Read the model definition and answer for the solid it produces. Units are mm, in the model's axes. A direction names the side the tool comes from. Give positions to 0.01 mm unless a question says otherwise; leave off trailing zeros. Order: outer loops, then holes, each group sorted by start corner. A loop starts at its lowest first (then second) coordinate and runs counter-clockwise, first axis right, second up. Notation, with made-up numbers: M 46,-39 L 75,-39 A12 cw 75,-32 Z; hole C 66.5,33 d7. An arc over 180 degrees is marked long. One line per item, written item: value.
from build123d import *

# Parameters (mm, degrees)
SKETCH_1_R          = 1.5
EXTRUDE_2_DEPTH     = 3
SKETCH_2_R          = 1.5
CUT_EXTRUDE_1_DEPTH = 10
CUT_EXTRUDE_2_DEPTH = 10


with BuildPart() as part:
    # 草图1 → 凸台-拉伸2 (new body)
    with BuildSketch(Plane(origin=(0, 0, 0), x_dir=(1, 0, 0), z_dir=(0, 1, 0))):
        with BuildLine():
            Line((-60, 65), (60, 65))
            ThreePointArc((60, 65), (125, 0), (60, -65))
            Line((60, -65), (-60, -65))
            ThreePointArc((-60, -65), (-125, 0), (-60, 65))
        make_face()
        with Locations((-122, 0)):
            Circle(SKETCH_1_R, mode=Mode.SUBTRACT)
        with Locations((122, 0)):
            Circle(SKETCH_1_R, mode=Mode.SUBTRACT)
        with Locations((-30, 60)):
            Circle(SKETCH_1_R, mode=Mode.SUBTRACT)
        with Locations((30, 60)):
            Circle(SKETCH_1_R, mode=Mode.SUBTRACT)
        with Locations((30, -60)):
            Circle(SKETCH_1_R, mode=Mode.SUBTRACT)
        with Locations((-30, -60)):
            Circle(SKETCH_1_R, mode=Mode.SUBTRACT)
    extrude(amount=EXTRUDE_2_DEPTH)

    # 草图2 → 切除-拉伸1 (cut)
    with BuildSketch(Plane(origin=(0, 3, 0), x_dir=(1, 0, 0), z_dir=(0, 1, 0))):
        with Locations((-10, 44)):
            Circle(SKETCH_2_R)
        with Locations((12, 44)):
            Circle(SKETCH_2_R)
        with Locations((-10, -44)):
            Circle(SKETCH_2_R)
        with Locations((12, -44)):
            Circle(SKETCH_2_R)
    extrude(amount=-CUT_EXTRUDE_1_DEPTH, mode=Mode.SUBTRACT)

    # 草图3 → 切除-拉伸2 (cut)
    with BuildSketch(Plane(origin=(0, 3, 0), x_dir=(1, 0, 0), z_dir=(0, 1, 0))):
        with BuildLine():
            Line((-77.5, 39), (77.5, 39))
            ThreePointArc((77.5, 39), (116.5, 0), (77.5, -39))
            Line((77.5, -39), (-77.5, -39))
            ThreePointArc((-77.5, -39), (-116.5, 0), (-77.5, 39))
        make_face()
    extrude(amount=-CUT_EXTRUDE_2_DEPTH, mode=Mode.SUBTRACT)


solid = part.part
1) Which of the six approach directions +Z, -Z, +X, -X, +Y, -Y give full straight-line access (tool end or side, diameter ignored) to faces 1 (the face through (116.49, 1.52, -0.86)), 2 (the face through (2, 3, 42))?
Reported:
face 1: +Y, -Y
face 2: +Z, -Z, +X, -X, +Y
2) This flat-tipped pin is pushed along its axis until it touches: pin 1 Ø1 at (y, z) = (2.5, -14.5) entering from -X. Where does it stop, or does it pass through?
Reported:
pin 1: stops at x = -123.47
3) Find section B-B, the plane y = 0.8. Count the separate pieces of the cut face and the enclosed holes in it, plus the area to 3 significant figures.
Reported:
separate pieces: 1
enclosed holes: 11
area: 11,900 mm^2
4) Find section A-A, the plane x = 36.5. Write down the section's boundary in (y, z).
Reported:
outline: M 0,-65 L 3,-65 L 3,-39 L 0,-39 Z; M 0,39 L 3,39 L 3,65 L 0,65 Z
5) Find section C-C, the plane z = -28.5. Write down the section's boundary in (x, y).
Reported:
outline: M -118.42,0 L -104.12,0 L -104.12,3 L -118.42,3 Z; M 104.12,0 L 118.42,0 L 118.42,3 L 104.12,3 Z
6) Determine the mould class of faces 3 (the face through (-116.49, 1.52, 0.86)), 4 (the face through (-124.984, 1.479, 1.429)), 5 (the face through (2, 0, 42)) for opening direction X: +X half, -X half, draft (parallel to the pull), parting line (faces both ways), or undercut.
Reported:
face 3: undercut
face 4: -X half
face 5: draft
7) Consider probe 1 along Z at (x, y) = (-30, 1.35); probe 2 along Z at (x, y) = (-10, 0.75); probe 3 along X at (y, z) = (2.3, 44). Determine where each line is inside the solid, lowest interval first.
Reported:
probe 1: z = -65 to -61.5, -58.5 to -39, 39 to 58.5, 61.5 to 65
probe 2: z = -65 to -45.5, -42.5 to -39, 39 to 42.5, 45.5 to 65
probe 3: x = -107.84 to -11.5, -8.5 to 10.5, 13.5 to 107.84
